```python
from build123d import *

# Parameters (mm, degrees)
SKETCH1_W           = 25.2
SKETCH1_H           = 25.2
SKETCH1_R           = 3.429
BOSS_EXTRUDE1_DEPTH = 4.6
SKETCH2_W           = 4.6
SKETCH2_H           = 25.2
BOSS_EXTRUDE2_DEPTH = 25.2
CUT_EXTRUDE1_REACH  = 46.13
SKETCH3_R           = 3.429
FILLET1_R           = 5


with BuildPart() as part:
    # Sketch1 → Boss-Extrude1 (new body)
    with BuildSketch(Plane(origin=(0, 0, 0), x_dir=(1, 0, 0), z_dir=(0, 1, 0))):
        with Locations((12.6, 12.6)):
            Rectangle(SKETCH1_W, SKETCH1_H)
        with Locations(Location((12.6, 12.6, 0), (0, 0, 270))):
            Circle(SKETCH1_R, mode=Mode.SUBTRACT)
    extrude(amount=BOSS_EXTRUDE1_DEPTH)

    # Sketch2 → Boss-Extrude2 (add)
    with BuildSketch(Plane(origin=(0, 4.6, 0), x_dir=(1, 0, 0), z_dir=(0, 1, 0))):
        with Locations((2.3, 12.6)):
            Rectangle(SKETCH2_W, SKETCH2_H)
    extrude(amount=BOSS_EXTRUDE2_DEPTH)

    # Sketch3 → Cut-Extrude1 (cut, up to next)
    with BuildSketch(Plane(origin=(4.6, 0, 0), x_dir=(0, 0, -1), z_dir=(1, 0, 0)), mode=Mode.PRIVATE) as cut_extrude1_sk1:
        with Locations((12.6, 14.9)):
            Circle(SKETCH3_R)
    cut_extrude1_tool1 = extrude(cut_extrude1_sk1.sketch, amount=-CUT_EXTRUDE1_REACH, mode=Mode.PRIVATE) & part.part
    add(cut_extrude1_tool1.solids().sort_by_distance((4.6, 14.9, -12.6))[0], mode=Mode.SUBTRACT)

    # Fillet1
    # the kernel refuses this fillet: 5 mm, written as the material it takes off along each edge
    with BuildSketch(Plane(origin=(4.6, 29.8, -37.659935794), x_dir=(-1, 0, 0), z_dir=(0, 0, 1))) as fillet1_piece_1:
        with BuildLine():
            CenterArc((5, 4.983974318), FILLET1_R, 180, 85.411434264)
            Line((0, 4.983974318), (-0.1, 4.983974318))
            Line((-0.1, 4.983974318), (-0.1, 0))
            Line((-0.1, 0), (0, -0.1))
            ThreePointArc((0, -0.1), (2.3, -0.1), (4.592, -0.099679486))
            Line((4.592, -0.099679486), (4.6, 0))
        make_face()
    extrude(amount=50.119871589, mode=Mode.SUBTRACT)
    with BuildSketch(Plane(origin=(25.2, 4.6, 12.459935794), x_dir=(-1, 0, 0), z_dir=(0, 0, -1))) as fillet1_piece_2:
        with BuildLine():
            CenterArc((4.983974318, -5), FILLET1_R, 90, 85.411434264)
            Line((0, -4.6), (-0.099679486, -4.592))
            ThreePointArc((-0.099679486, -4.592), (-0.1, -2.3), (-0.1, 0))
            Line((-0.1, 0), (0, 0.1))
            Line((0, 0.1), (4.983974318, 0.1))
            Line((4.983974318, 0.1), (4.983974318, 0))
        make_face()
    extrude(amount=50.119871589, mode=Mode.SUBTRACT)


solid = part.part
```
Here's how the part is built. I have some questions about the finished solid (model axes, mm). A direction names the side the tool comes from. Coordinates: 2 decimals unless noted, no trailing zeros. Order: outer loops, then holes, each group sorted by start corner. A loop starts at its lowest first (then second) coordinate and runs counter-clockwise, first axis right, second up. Notation, with made-up numbers: M -4,26 L 43,26 A11 cw 43,38 Z; hole C 38.25,-37 d8. An arc over 180 degrees is marked long. Answer as a JSON object with one key per item and string values. Group by question number.
(1) Suppose I cut it at B-B, the plane z = -12.6. Please give me the cut outline in (x, y), then the cut area to 3 significant figures.
(2) Suppose I cut it at A-A, the plane x = 12.6. Please give me the cut outline in (y, z), then the cut area to 3 significant figures.
(3) Suppose I cut it at D-D, the plane z = -22.75. Please give me the cut outline in (x, y).
(4) If we mould it in two halves opening along Z, with no side actions, what happens to faces 1 (the face through (11.29, 2.27, -9.43)), 2 (the face through (23.57, 3.31, -12.42)), 3 (the face through (4, 8, -25.2))? For each: released by +Z, released by -Z, zero draft, split by the parting line, or undercut.
(5) For pin 1 (1.5 mm diameter, centred on y = 6.5, z = -12.5, fed in from +X); pin 2 (6 mm diameter, centred on y = 5, z = -4, fed in from +X); pin 3 (4.5 mm diameter, centred on x = 13, z = -18, fed in from +Y), each with a flat end and sliding along its axis, tell me the tip position at first contact or that it passes through.
(6) I need wall thicknesses on probe 1 along X at (y, z) = (12, -17.75); probe 2 along Y at (x, z) = (1.15, -12.6). Which ranges of each line are inside material? Lowest first, please.
(7) Which directions (+Z, -Z, +X, -X, +Y, -Y) give clear straight access to the entire face, cutting with the end or side of a thin tool? Please do faces 4 (the face through (0, 11, -12)), 5 (the face through (11, 4.6, -16)).
Values found:
{
 "1": {"outline": "M 0,0 L 9.17,0 L 9.17,4.6 L 4.6,4.6 L 4.6,11.47 L 0,11.47 Z; M 0,18.33 L 4.6,18.33 L 4.6,24.82 A5 ccw 0,29.8 Z; M 16.03,0 L 25.2,0 A5 ccw 20.22,4.6 L 16.03,4.6 Z", "area": "158 mm^2"},
 "2": {"outline": "M 0,-25.2 L 4.6,-25.2 L 4.6,-16.03 L 0,-16.03 Z; M 0,-9.17 L 4.6,-9.17 L 4.6,0 L 0,0 Z", "area": "84.4 mm^2"},
 "3": {"outline": "M 0,0 L 25.2,0 A5 ccw 20.22,4.6 L 4.6,4.6 L 4.6,24.82 A5 ccw 0,29.8 Z"},
 "4": {"face 1": "undercut", "face 2": "zero draft", "face 3": "released by -Z"},
 "5": {"pin 1": "stops at x = 4.6", "pin 2": "stops at x = 24.6", "pin 3": "stops at y = 4.6"},
 "6": {"probe 1": "x = 0 to 4.6", "probe 2": "y = 0 to 11.47, 18.33 to 29.57"},
 "7": {"face 4": "+Z, -Z, -X, +Y, -Y", "face 5": "+Z, -Z, +X, +Y"}
}
